Autodesk Inventor part; units mm, degrees
ref_plane "YZ Plane" through (0, 0, 0) normal (1, 0, 0) x (0, 1, 0)
ref_plane "XZ Plane" through (0, 0, 0) normal (0, 1, 0) x (-1, 0, 0)
ref_plane "XY Plane" through (0, 0, 0) normal (0, 0, 1) x (1, 0, 0)
sketch "Boceto1" plane through (0, 0, 0) normal (0, 1, 0) x (-1, 0, 0)
  line L0 (0, 0) -> (60, 0)
  line L1 (60, 0) -> (60, 60)
  line L2 (60, 60) -> (0, 60)
  line L3 (0, 60) -> (0, 0)
  line L4 (3, 57) -> (57, 57)
  line L5 (57, 57) -> (57, 3)
  line L6 (57, 3) -> (3, 3)
  line L7 (3, 3) -> (3, 57)
  line L8 (-3, 63) -> (63, 63)
  line L9 (63, 63) -> (63, -3)
  line L10 (63, -3) -> (-3, -3)
  line L11 (-3, -3) -> (-3, 63)
  dimension "d0" = 60
  dimension "d1" = 60
  dimension "d3" = 3
  dimension "d13" = 3
extrude "Extrusión1" add sketch "Boceto1" along normal blind 6 contours L8 L9 L10 L11
sketch "Boceto2" plane through (0, 0, 0) normal (0, -1, 0) x (1, 0, 0)
  line L0 (3, -3) -> (-63, -3)
  line L1 (3, 63) -> (3, -3)
  line L2 (-63, 63) -> (3, 63)
  line L3 (-63, -3) -> (-63, 63)
  line L4 (0, 0) -> (0, 60)
  line L5 (-60, 0) -> (0, 0)
  line L6 (-60, 60) -> (-60, 0)
  line L7 (0, 60) -> (-60, 60)
extrude "Extrusión2" add sketch "Boceto2" along normal blind 2 contours L0 L3 L2 L1 | L5 L6 L7 L4
sketch "Boceto3" plane through (0, 6, 0) normal (0, 1, 0) x (1, 0, 0)
  line L0 (0, 0) -> (0, -60)
  line L1 (0, -60) -> (3, -60)
  line L2 (3, -60) -> (3, 0)
  line L3 (3, 0) -> (0, 0)
  line L4 (0, 0) -> (0, -60)
extrude "Extrusión3" cut sketch "Boceto3" against normal up to surface (6 mm away)
sketch "Boceto4" plane through (0, 0, 0) normal (0, 1, 0) x (1, 0, 0)
  line L0 (-60, 0) -> (3, 0)
  line L1 (-60, -60) -> (-60, 0)
  line L2 (-60, -60) -> (3, -60)
  line L3 (3, 0) -> (3, -60)
  line L4 (3, -60) -> (0, -60)
  line L5 (0, -60) -> (0, 0)
  line L6 (0, -57) -> (0, -3)
  line L7 (0, -3) -> (-57, -3)
  line L8 (-57, -3) -> (-57, -57)
  line L9 (-57, -57) -> (0, -57)
  line L10 (-3, 0) -> (-3, -63)
  line L11 (-3, -63) -> (3, -63)
  point P0 (-3, -57)
  point P1 (-3, -3)
  dimension "d28" = 3
extrude "Extrusión4" cut sketch "Boceto4" against normal blind 10 contours L10 L9 L8 L7
fillet "Empalme1" radius 10 4 edges at (-3, -1, 57) (-3, -1, 3) (-57, -1, 3) (-57, -1, 57)
properties part number "Disco_inferior"
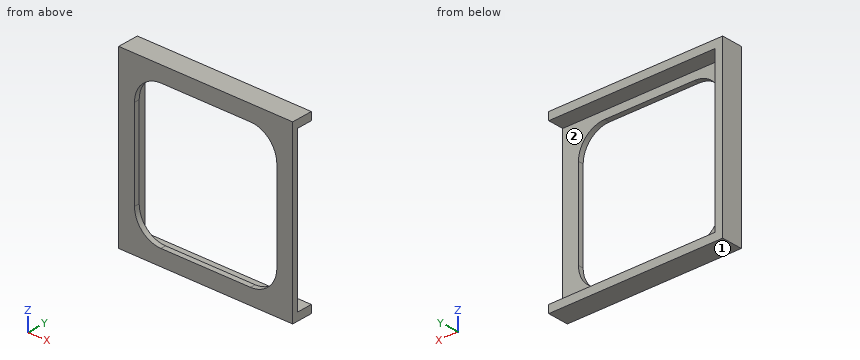
Model file for the job. Use its own axes, mm. Face numbers are marked on the shaded views. A direction names the side the tool comes from. Round coordinates to 2 decimals unless told otherwise and drop trailing zeros. Write each loop counter-clockwise with the first axis right and the second up, starting at its lowest first coordinate (ties: lowest second). Pieces come first, ordered by that corner, then holes. Notation, with made-up numbers: (13.25, 60) -> (20.25, 60) arc R22 cw to (20.25, 73) -> close; hole circle Ø3 at (7.25, 35). An arc over 180 degrees is marked (long way). Answer as CSV lines item,"result".
1. Slice it at B-B, the plane x = -26. List the corners of the cut face in (y, z).
Resolved:
outline,"(-2, -3) -> (6, -3) -> (6, 0) -> (0, 0) -> (0, 3) -> (-2, 3) -> close; (-2, 57) -> (0, 57) -> (0, 60) -> (6, 60) -> (6, 63) -> (-2, 63) -> close"
2. Tool access for the marked faces 1 and 2: list every direction of +Z, -Z, +X, -X, +Y, -Y with a clear straight run to the whole face (end or side of a thin tool).
Resolved:
face 1,"-Z, +X, -X, +Y, -Y"
face 2,"+X, +Y"
3. Drill centre lines: line 1 (Z direction, x = -17, y = 4.5); line 2 (X direction, y = 3.5, z = 16); line 3 (Z direction, x = -12.5, y = -0.75). Where is each one in solid material? Low to high.
Resolved:
line 1,"-3 to 0, 60 to 63"
line 2,"-63 to -60"
line 3,"-3 to 3.01, 56.99 to 63"
4. Pin check, flat tip, straight feed: pin 1 Ø3 at (y, z) = (2.5, 26.5) entering from +X. Stop position of the tip, or through.
Resolved:
pin 1,"x = -60"
5. Slice it at C-C, the plane x = -1.5. List the corners of the cut face in (y, z).
Resolved:
outline,"(-2, -3) -> (6, -3) -> (6, 0) -> (0, 0) -> (0, 60) -> (6, 60) -> (6, 63) -> (-2, 63) -> close"
6. Slice it at A-A, the plane z = 35. List the corners of the cut face in (x, y), plus the area to 3 significant figures.
Resolved:
outline,"(-63, -2) -> (-57, -2) -> (-57, 0) -> (-60, 0) -> (-60, 6) -> (-63, 6) -> close; (-3, -2) -> (3, -2) -> (3, 0) -> (-3, 0) -> close"
area,"42.0 mm²"
7. Slice it at D-D, the plane y = 4.5. List the corners of the cut face in (x, z).
Resolved:
outline,"(-63, -3) -> (3, -3) -> (3, 0) -> (-60, 0) -> (-60, 60) -> (3, 60) -> (3, 63) -> (-63, 63) -> close"
